from build123d import *

# Parameters (mm, degrees)
SKETCH1_W             = 10
SKETCH1_H             = 32
SKETCH1_R             = 2.4
BOSS_EXTRUDE1_DEPTH   = 7
BOSS_EXTRUDE1_2_DEPTH = 7
SKETCH3_R             = 1.6
BOSS_EXTRUDE2_DEPTH   = 2
SKETCH2_R             = 3.5
CUT_EXTRUDE2_DEPTH    = 6
SKETCH4_W             = 40
SKETCH4_H             = 40
CUT_EXTRUDE3_DEPTH    = 47.238512087
FILLET1_R             = 2
CHAMFER1_SIZE         = 2


with BuildPart() as part:
    # Sketch1 → Boss-Extrude1 (new, symmetric)
    with BuildSketch(Plane.XY):
        with Locations((-32, 0)):
            Rectangle(SKETCH1_W, SKETCH1_H)
        with Locations((-32, 0)):
            Circle(SKETCH1_R, mode=Mode.SUBTRACT)
    extrude(amount=BOSS_EXTRUDE1_DEPTH, both=True)



with BuildPart() as body_2:
    # Sketch1 → Boss-Extrude1 2 (new, symmetric)
    with BuildSketch(Plane.XY):
        with Locations((32, 0)):
            Rectangle(SKETCH1_W, SKETCH1_H)
        with Locations((32, 0)):
            Circle(SKETCH1_R, mode=Mode.SUBTRACT)
    extrude(amount=BOSS_EXTRUDE1_2_DEPTH, both=True)


with BuildPart() as part_1:
    add(part.part)

    add(body_2.part)  # Boss-Extrude2 merges body 2
    # Sketch3 → Boss-Extrude2 (add)
    with BuildSketch(Plane.XY.offset(7)):
        Polygon((-37, 16), (-30, 16), (-30, 25), (30, 25), (30, 16), (37, 16), (37, -16), (30, -16), (30, -25), (-30, -25), (-30, -16), (-37, -16), align=None)
        with Locations((-25, 20)):
            Circle(SKETCH3_R, mode=Mode.SUBTRACT)
        with Locations((25, 20)):
            Circle(SKETCH3_R, mode=Mode.SUBTRACT)
        with Locations((25, -20)):
            Circle(SKETCH3_R, mode=Mode.SUBTRACT)
        with Locations((-25, -20)):
            Circle(SKETCH3_R, mode=Mode.SUBTRACT)
    extrude(amount=-BOSS_EXTRUDE2_DEPTH)

    # Sketch2 → Cut-Extrude2 (cut)
    with BuildSketch(Plane.XY.offset(7)):
        with Locations((-32, 0)):
            Circle(SKETCH2_R)
        with Locations((32, 0)):
            Circle(SKETCH2_R)
        with Locations((-25, 20)):
            Circle(SKETCH2_R)
        with Locations((25, 20)):
            Circle(SKETCH2_R)
        with Locations((25, -20)):
            Circle(SKETCH2_R)
        with Locations((-25, -20)):
            Circle(SKETCH2_R)
    extrude(amount=-CUT_EXTRUDE2_DEPTH, mode=Mode.SUBTRACT)

    # Sketch4 → Cut-Extrude3 (cut, through all)
    with BuildSketch(Plane(origin=(0, 0, 5), x_dir=(-1, 0, 0), z_dir=(0, 0, -1))):
        with Locations((0, -5)):
            Rectangle(SKETCH4_W, SKETCH4_H)
    extrude(amount=-CUT_EXTRUDE3_DEPTH, mode=Mode.SUBTRACT)

    # Fillet1
    fillet1_edges = [part_1.edges().sort_by_distance(p)[0] for p in [
        (20, -25, 6),
        (20, 15, 6),
        (-20, 15, 6),
        (-20, -25, 6),
        (-27, 16, -1),
        (-27, -16, -1),
        (-30, 16, 6),
        (-30, 25, 6),
        (30, 25, 6),
        (30, 16, 6),
        (37, 16, 0),
        (37, -16, 0),
        (30, -16, 6),
        (30, -25, 6),
        (-30, -25, 6),
        (-30, -16, 6),
        (27, 16, -1),
        (27, -16, -1),
        (-37, 16, 0),
        (-37, -16, 0),
    ]]
    fillet(fillet1_edges, radius=FILLET1_R)

    # Chamfer1
    # the kernel refuses this chamfer: 2 mm, written as the material it takes off along each edge
    with BuildSketch(Plane(origin=(-32, 0, 1), x_dir=(1, 0, 0), z_dir=(0, 1, 0))) as chamfer1_piece_1_section:
        Polygon((2.4 + CHAMFER1_SIZE, 0), (2.4, CHAMFER1_SIZE), (2.4, 0), align=None)
    chamfer1_piece_1 = revolve(axis=Axis((-32, 0, 1), (0, 0, -1)), mode=Mode.PRIVATE)
    chamfer1_piece_1 = chamfer1_piece_1 & Plane(origin=(-32, 0, -0.456047854), x_dir=(1, 0, 0), z_dir=(0, 0, 1)) * Cylinder(3.5, 18, mode=Mode.PRIVATE)
    add(chamfer1_piece_1, mode=Mode.SUBTRACT)
    with BuildSketch(Plane(origin=(32, 0, 1), x_dir=(1, 0, 0), z_dir=(0, 1, 0))) as chamfer1_piece_2_section:
        Polygon((2.4, CHAMFER1_SIZE), (2.4 + CHAMFER1_SIZE, 0), (2.4, 0), align=None)
    chamfer1_piece_2 = revolve(axis=Axis((32, 0, 1), (0, 0, -1)), mode=Mode.PRIVATE)
    chamfer1_piece_2 = chamfer1_piece_2 & Plane(origin=(32, 0, -0.456047854), x_dir=(1, 0, 0), z_dir=(0, 0, 1)) * Cylinder(3.5, 18, mode=Mode.PRIVATE)
    add(chamfer1_piece_2, mode=Mode.SUBTRACT)


solid = part_1.part
Input: part model. Units: mm. Frame: model coordinates. A direction names the side the tool comes from. Round coordinates to 2 decimals unless told otherwise and drop trailing zeros. Order: outer loops, then holes, each group sorted by start corner. A loop starts at its lowest first (then second) coordinate and runs counter-clockwise, first axis right, second up. Notation, with made-up numbers: (77.25, 23) - (102.25, 23) arc R22 cw to (102.25, 55) - close; hole circle Ø5 at (10.25, 65). An arc over 180 degrees is marked (long way). Answer as a JSON object with one key per item and string values. Group by question number.
(1) Cut plane C-C (x = -25). Return loops of the section in (y, z), then the cut area to 3 significant figures.
(2) Cut plane D-D (y = 20). Return loops of the section in (x, z), then the cut area to 3 significant figures.
(3) Reachability of faces 4 (the face through (-30, -21, 6)), 5 (the face through (-30, 20, 6)), 6 (the face through (30, -20, 6)) from +Z, -Z, +X, -X, +Y, -Y: full face, straight path, thin tool, end or side. Return the list, or none.
(4) Cut plane A-A (z = 3.25). Return loops of the section in (x, y), then the cut area to 3 significant figures.
(5) Draft query along Y for faces 1 (the face through (-30.6, -16.57, 5.99)), 2 (the face through (-23.12, 22.95, 6.01)), 3 (the face through (29.4, 24.43, 5.99)). Return one class per face: released by +Y, released by -Y, zero draft, split by the parting line, or undercut.
(6) Cut plane B-B (y = -12). Return loops of the section in (x, z), then the cut area to 3 significant figures.
(7) Pin query (flat end, axial travel): P1, Ø6.5, axis at x = -25, y = -20, coming from the +Z side; P2, Ø5, axis at x = 28, z = -1.5, coming from the +Y side; P3, Ø6.5, axis at x = 32.5, z = 2, coming from the -Y side; P4, Ø1.6, axis at y = 20.5, z = 6.5, coming from the -X side. Return the tip coordinate at first contact, or that it passes through.
(8) Material intervals for probe 1 along Y at (x, z) = (25, 5.55); probe 2 along X at (y, z) = (0, -3.5); probe 3 along Y at (x, z) = (32, 4.75), sorted ascending. Write a range as from..to.
Here are the results:
{
 "1": {"outline": "(-25, 5) - (-23.5, 5) - (-23.5, 7) - (-25, 7) - close; (-16.5, 5) - (16.5, 5) - (16.5, 7) - (-16.5, 7) - close; (23.5, 5) - (25, 5) - (25, 7) - (23.5, 7) - close", "area": "72.0 mm^2"},
 "2": {"outline": "(-30, 5) - (-28.5, 5) - (-28.5, 7) - (-30, 7) - close; (-21.5, 5) - (21.5, 5) - (21.5, 7) - (-21.5, 7) - close; (28.5, 5) - (30, 5) - (30, 7) - (28.5, 7) - close", "area": "92.0 mm^2"},
 "3": {"face 4": "+Z, -Z, -X, -Y", "face 5": "+Z, -Z, -X, +Y", "face 6": "+Z, -Z, +X, -Y"},
 "4": {"outline": "(-37, -14) arc R2 ccw to (-35, -16) - (-29, -16) arc R2 ccw to (-27, -14) - (-27, 14) arc R2 ccw to (-29, 16) - (-35, 16) arc R2 ccw to (-37, 14) - close; (27, -14) arc R2 ccw to (29, -16) - (35, -16) arc R2 ccw to (37, -14) - (37, 14) arc R2 ccw to (35, 16) - (29, 16) arc R2 ccw to (27, 14) - close; hole circle Ø7 at (-32, 0); hole circle Ø7 at (32, 0)", "area": "556 mm^2"},
 "5": {"face 1": "released by -Y", "face 2": "undercut", "face 3": "released by +Y"},
 "6": {"outline": "(-37, -7) - (-27, -7) - (-27, 5) - (-20, 5) - (-20, 7) - (-37, 7) - close; (20, 5) - (27, 5) - (27, -7) - (37, -7) - (37, 7) - (20, 7) - close", "area": "308 mm^2"},
 "7": {"P1": "passes through", "P2": "stops at y = 16", "P3": "stops at y = -16.15", "P4": "stops at x = -30"},
 "8": {"probe 1": "y = -25..-23.5, -16.5..16.5, 23.5..25", "probe 2": "x = -37..-34.4, -29.6..-27, 27..29.6, 34.4..37", "probe 3": "y = -16..-3.5, 3.5..16"}
}
